Autodesk Inventor part; units mm, degrees
ref_plane "YZ Plane" through (0, 0, 0) normal (1, 0, 0) x (0, 1, 0)
ref_plane "XZ Plane" through (0, 0, 0) normal (0, 1, 0) x (-1, 0, 0)
ref_plane "XY Plane" through (0, 0, 0) normal (0, 0, 1) x (1, 0, 0)
sketch "Sketch1" plane through (0, 0, 0) normal (0, 1, 0) x (-1, 0, 0)
  line L0 (13.125, 9.625) -> (-13.125, 9.625)
  line L1 (-13.125, 9.625) -> (-13.125, -9.625)
  line L2 (-13.125, -9.625) -> (13.125, -9.625)
  line L3 (13.125, -9.625) -> (13.125, 9.625)
  line L4 (13.125, 9.625) -> (-13.125, -9.625) construction
  line L5 (-13.125, 9.625) -> (13.125, -9.625) construction
  circle A0 centre (8.625, -6.925) radius 1.5
  circle A1 centre (-8.625, -6.925) radius 1.5
  line L6 (3.375, 7.625) -> (-8.825, 7.625)
  line L7 (-8.825, 7.625) -> (-8.825, -4.225)
  line L8 (-8.825, -4.225) -> (3.375, -4.225)
  line L9 (3.375, -4.225) -> (3.375, 7.625)
  line L10 (3.375, 7.625) -> (-8.825, -4.225) construction
  line L11 (-8.825, 7.625) -> (3.375, -4.225) construction
  point P0 (0, 0)
  point P1 (-2.725, 1.7)
  dimension "d0" = 26.25
  dimension "d1" = 19.25
  dimension "d2" = 3
  dimension "d3" = 3
  dimension "d5" = 2.7
  dimension "d8" = 4.5
  dimension "d9" = 4.5
  dimension "d11" = 2.7
  dimension "d12" = 12.2
  dimension "d13" = 11.85
  dimension "d14" = 2
  dimension "d15" = 4.3
extrude "Extrusion1" add sketch "Sketch1" against normal blind 1.5
sketch "Sketch2" plane through (0, -1.5, 0) normal (0, -1, 0) x (1, 0, 0)
  line L0 (8.825, -4.225) -> (8.825, 7.625)
  line L1 (8.825, 7.625) -> (-3.375, 7.625)
  line L2 (-3.375, 7.625) -> (-3.375, -4.225)
  line L3 (-3.375, -4.225) -> (8.825, -4.225)
  circle A0 centre (8.625, -6.925) radius 1.5
  circle A1 centre (-8.625, -6.925) radius 1.5
  line L4 (-13.125, 9.625) -> (13.125, 9.625)
  line L5 (13.125, 9.625) -> (13.125, -9.625)
  line L6 (13.125, -9.625) -> (-13.125, -9.625)
  line L7 (-13.125, -9.625) -> (-13.125, 9.625)
  point P0 (0, 0)
extrude "Extrusion2" add sketch "Sketch2" against normal blind 8.12 contours L3 L2 L1 L0
sketch "Sketch3" plane through (0, 0, 0) normal (0, 1, 0) x (1, 0, 0)
  line L0 (-18.725, -8.875) -> (-8.725, -8.875)
  line L1 (-8.725, -8.875) -> (-8.725, 3.525)
  line L2 (-8.725, 3.525) -> (-18.725, 3.525)
  line L3 (-18.725, 3.525) -> (-18.725, -8.875)
  line L4 (-18.725, -8.875) -> (-8.725, 3.525) construction
  line L5 (-8.725, -8.875) -> (-18.725, 3.525) construction
  line L6 (-13.125, 9.625) -> (-13.125, -9.625)
  line L7 (13.125, 9.625) -> (-13.125, 9.625)
  point P0 (0, 0)
  point P1 (-13.725, -2.675)
  dimension "d20" = 10
  dimension "d21" = 12.4
  dimension "d22" = 4.4
  dimension "d23" = 18.5
extrude "Extrusion3" add sketch "Sketch3" along normal blind 4.5
sketch "Sketch4" plane through (0, 6.62, 0) normal (0, 1, 0) x (1, 0, 0)
  line L0 (8.825, -7.625) -> (8.825, 4.225)
  line L1 (8.825, 4.225) -> (-3.375, 4.225)
  line L2 (-3.375, 4.225) -> (-3.375, -7.625)
  line L3 (-3.375, -7.625) -> (8.825, -7.625)
  circle A0 centre (2.725, -1.7) radius 3.35
  point P0 (0, 0)
  dimension "d26" = 6.7
extrude "Extrusion4" add sketch "Sketch4" along normal blind 7.5 contours A0
sketch "Sketch5" plane through (2.725, 14.12, 1.7) normal (0, 1, 0) x (1, 0, 0)
  circle A0 centre (0, 0) radius 3.35
  circle A1 centre (0, 0) radius 3
  point P0 (-2.725, 1.7)
  dimension "d29" = 6
extrude "Extrusion5" add sketch "Sketch5" along normal blind 12.56 contours A1
sketch "Sketch6" plane through (2.725, 26.68, 1.7) normal (0, 1, 0) x (1, 0, 0)
  circle A0 centre (0, 0) radius 3
  line L0 (1.7, 2.4718) -> (1.7, -2.4718)
  point P0 (-2.725, 1.7)
  dimension "d32" = 1.7
extrude "Extrusion6" cut sketch "Sketch6" against normal blind 10 contours A0 L0 picked at (2.1333, 0)
fillet "Fillet1" radius 0.2 1 edges at (-0.275, 26.68, 1.7)
equation "\"d11\" = d5"
properties part number "encoder"
CAD build for the part. Positions are in the model's coordinates, mm. A direction names the side the tool comes from. Give positions to 0.01 mm unless a question says otherwise; leave off trailing zeros. Loops run counter-clockwise (first coordinate to the right, second up) from the corner with the lowest first, then second, coordinate; pieces in that order, holes last. Notation, with made-up numbers: (42, -29.5) - (71, -29.5) arc R30 cw to (71, -5.5) - close; hole circle Ø2 at (25.25, 53). An arc over 180 degrees is marked (long way). Put each result on its own line as item: value.
Q1. Tool access for faces 1 (the face through (0, 6.62, -1)), 2 (the face through (-3.375, 3, 2)), 3 (the face through (8.825, 3, 2)), 4 (the face through (-13.125, -1, 0)), 5 (the face through (-14, 2, 8.875)): list every direction of +Z, -Z, +X, -X, +Y, -Y with a clear straight run to the whole face (end or side of a thin tool).
Filled in:
face 1: +Y
face 2: +Z, -Z, +Y
face 3: +Z, -Z, +X, +Y
face 4: +Z, -Z, -X, -Y
face 5: +Z, +X, -X, +Y
Q2. Slice it at A-A (y = 3). Give the cut face in (x, z) (3 decimals), plus the area to 3 significant figures.
Filled in:
outline: (-18.725, -3.525) - (-8.725, -3.525) - (-8.725, 8.875) - (-18.725, 8.875) - close; (-3.375, -4.225) - (8.825, -4.225) - (8.825, 7.625) - (-3.375, 7.625) - close
area: 269 mm²
Q3. Probe line 1 along Y through (x, z) = (12, 5.5); line 2 along X through (y, z) = (3.25, -1) (3 decimals); line 3 along Y through (x, z) = (7, 5.75). List the from-to ranges inside material, lowest first.
Filled in:
line 1: y = -1.5 to 0
line 2: x = -18.725 to -8.725, -3.375 to 8.825
line 3: y = -1.5 to 6.62
Q4. Slice it at D-D (y = 14.75). Give the cut face in (x, z) (3 decimals), plus the area to 3 significant figures.
Filled in:
outline: circle Ø6 at (2.725, 1.7)
area: 28.3 mm²
Q5. Slice it at C-C (x = -1.5). Give the cut face in (y, z) (3 decimals).
Filled in:
outline: (-1.5, -9.625) - (0, -9.625) - (0, -4.225) - (6.62, -4.225) - (6.62, 7.625) - (0, 7.625) - (0, 9.625) - (-1.5, 9.625) - close
Q6. Slice it at B-B (z = 6.75). Give the cut face in (x, y) (3 decimals), plus the area to 3 significant figures.
Filled in:
outline: (-18.725, 0) - (-13.125, 0) - (-13.125, -1.5) - (13.125, -1.5) - (13.125, 0) - (8.825, 0) - (8.825, 6.62) - (-3.375, 6.62) - (-3.375, 0) - (-8.725, 0) - (-8.725, 4.5) - (-18.725, 4.5) - close
area: 165 mm²
Q7. Flat gauge pins, fed straight in: pin 1 (4 mm diameter, centred on x = 8.625, z = -6.925, fed in from -Y); pin 2 (4.5 mm diameter, centred on x = -17, z = 1, fed in from -Y); pin 3 (3 mm diameter, centred on y = 23, z = 3.5, fed in from +X) (3 decimals); pin 4 (1.6 mm diameter, centred on y = -1, z = 1.5, fed in from -X) (3 decimals). Where does each tip first touch, or does it go through?
Filled in:
pin 1: stops at y = -1.5
pin 2: stops at y = 0
pin 3: stops at x = 4.425
pin 4: stops at x = -13.125
